Autodesk Inventor part; units mm, degrees
ref_plane "YZ Plane" through (0, 0, 0) normal (1, 0, 0) x (0, 1, 0)
ref_plane "XZ Plane" through (0, 0, 0) normal (0, 1, 0) x (-1, 0, 0)
ref_plane "XY Plane" through (0, 0, 0) normal (0, 0, 1) x (1, 0, 0)
sketch "Sketch1" plane through (0, 0, 0) normal (0, 0, 1) x (1, 0, 0)
  circle A0 centre (0, 0) radius 2.5
  line L0 (-8, 5) -> (8, 5)
  line L1 (9, 4) -> (9, -4)
  line L2 (8, -5) -> (-8, -5)
  line L3 (-9, -4) -> (-9, 4)
  line L4 (-8, 5) -> (-9, 4)
  line L5 (-9, -4) -> (-8, -5)
  line L6 (8, -5) -> (9, -4)
  line L7 (9, 4) -> (8, 5)
  point P0 (-9, 5)
  point P1 (9, -5)
  point P2 (9, 5)
  point P3 (-9, -5)
  point P4 (0, 5)
  point P5 (9, 0)
  dimension "d0" = 5
  dimension "d1" = 1
  dimension "d2" = 1
  dimension "d3" = 1
  dimension "d4" = 1
  dimension "d5" = 1
  dimension "d6" = 1
  dimension "d7" = 1
  dimension "d8" = 1
  dimension "d9" = 18
  dimension "d10" = 10
extrude "Extrusion1" add sketch "Sketch1" along normal blind 7.2
properties part number "Slide"
Build history of the part. All positions in model axes, mm. Coordinates: 2 decimals unless noted, no trailing zeros. Write each loop counter-clockwise with the first axis right and the second up, starting at its lowest first coordinate (ties: lowest second). Pieces come first, ordered by that corner, then holes.
1. Band-saw the part on B-B, the plane z = 6.5. Give the cut face in (x, y), and give its area (3 significant figures).
Answer block:
outline: (-9, -4) - (-8, -5) - (8, -5) - (9, -4) - (9, 4) - (8, 5) - (-8, 5) - (-9, 4) - close; hole circle Ø5 at (0, 0)
area: 158 mm2
2. Pull direction X, two halves, no side cores. Call faces 1 (the flat face through (8.5, -4.5, 3.5)), 2 (the cylindrical face through (-0.54, 2.44, 3.55)), 3 (the flat face through (0, -5, 4)), 4 (the flat face through (-9, 0, 4)): released by +X, released by -X, zero draft, split by the parting line, or undercut.
Answer block:
face 1: released by +X
face 2: undercut
face 3: zero draft
face 4: released by -X
3. Drill centre lines: probe 1 along Y at (x, z) = (0, 2.5); probe 2 along Y at (x, z) = (-1, 5); probe 3 along X at (y, z) = (-2.25, 5.25). Where is each one in solid material? Low to high.
Answer block:
probe 1: y = -5 to -2.5, 2.5 to 5
probe 2: y = -5 to -2.29, 2.29 to 5
probe 3: x = -9 to -1.09, 1.09 to 9
4. Band-saw the part on A-A, the plane y = 0. Give the cut face in (x, z).
Answer block:
outline: (-9, 0) - (-2.5, 0) - (-2.5, 7.2) - (-9, 7.2) - close; (2.5, 0) - (9, 0) - (9, 7.2) - (2.5, 7.2) - close
5. Band-saw the part on C-C, the plane x = 1.5. Give the cut face in (y, z).
Answer block:
outline: (-5, 0) - (-2, 0) - (-2, 7.2) - (-5, 7.2) - close; (2, 0) - (5, 0) - (5, 7.2) - (2, 7.2) - close
